Autodesk Inventor part; units mm, degrees
ref_plane "YZ Plane" through (0, 0, 0) normal (1, 0, 0) x (0, 1, 0)
ref_plane "XZ Plane" through (0, 0, 0) normal (0, 1, 0) x (-1, 0, 0)
ref_plane "XY Plane" through (0, 0, 0) normal (0, 0, 1) x (1, 0, 0)
sketch "Block1" plane through (0, 0, 0) normal (0, 0, 1) x (1, 0, 0)
  circle A0 centre (40.64, 3.81) radius 3.81
  point P0 (32.0567, 3.81)
sketch "Sketch1" plane through (0, 0, 0) normal (0, 1, 0) x (-1, 0, 0)
  line L0 (5.08, 5.08) -> (-5.08, 5.08)
  line L1 (-5.08, 5.08) -> (-5.08, -39.37)
  line L2 (-5.08, -39.37) -> (5.08, -39.37)
  line L3 (5.08, -39.37) -> (5.08, 5.08)
  point P0 (0, 0)
  dimension "d0" = 10.16
  dimension "d1" = 44.45
extrude "bar" add sketch "Sketch1" along normal blind 7.62
sketch "Sketch2" plane through (-5.08, 0, -39.37) normal (-1, 0, 0) x (0, 0, 1)
  circle A0 centre (4, 3.81) radius 2.175
  circle A1 centre (16, 3.81) radius 2.175
  circle A2 centre (9.9822, 3.81) radius 1.0704
  point P0 (39.37, 0)
  dimension "d4" = 4.35
  dimension "d5" = 4.35
hole "pegholes" at (-5.08, 3.81, -35.37) at (-5.08, 3.81, -23.37) direction (1, 0, 0) diameter 4.35 end through all
fillet "Fillet3" radius 3.81 3 edges at (0, 7.62, -39.37) (0, 0, -39.37) (0, 7.62, 5.08)
sketch "Sketch3" plane through (5.08, 0, 5.08) normal (1, 0, 0) x (0, 0, -1)
  line L0 (40.64, 7.62) -> (3.81, 7.62)
  line L1 (23.6161, 7.62) -> (40.64, 7.62)
  line L2 (40.64, 7.62) -> (40.64, 0)
  line L3 (40.64, 0) -> (23.6161, 0)
  line L4 (23.6161, 0) -> (23.6161, 7.62)
  circle A0 centre (40.64, 3.81) radius 3.81
  point P0 (5.08, 0)
extrude "Extrusion2" cut sketch "Sketch3" against normal blind 5.334 contours A0 L2 | L2 A0
extrude "Extrusion3" cut sketch "Sketch3" against normal blind 5.334 contours A0 L3 L4 L0 | L2 A0 picked at (39.3793, 3.6569)
fillet "Fillet4" radius 5.334 1 edges at (5.08, 3.81, -18.5361)
properties part number "fire-bar"
Can you work these out from the model? Positions are in its coordinate system, mm. A direction names the side the tool comes from. Coordinates: 2 decimals unless noted, no trailing zeros. Loops run counter-clockwise (first coordinate to the right, second up) from the corner with the lowest first, then second, coordinate; pieces in that order, holes last.
1) Imagine slicing it at C-C on x = 1.5. List the corners of the cut face in (y, z) for me, plus the area to 3 significant figures.
2) Thinking about a two-plate mould opening in Y: for faces 3 (the flat face through (-1, 7.62, -13)), 4 (the flat face through (-1, 0, -10)), 5 (the cylindrical face through (-2.633, 3.157, -21.295)), 6 (the flat face through (-5.08, 4, -17)), which applies, pulls with the +Y half, pulls with the -Y half, needs draft (parallel to the pull), parting line crosses it, or undercut?
3) For pin 1 (4 mm diameter, centred on y = 3.5, z = -32, fed in from +X); pin 2 (3 mm diameter, centred on x = -2, y = 5.5, fed in from -Z), each with a flat end and sliding along its axis, tell me the tip position at first contact or that it passes through.
4) Imagine slicing it at D-D on z = -29.5. List the corners of the cut face in (x, y) for me, plus the area to 3 significant figures.
5) Imagine slicing it at A-A on z = -23.37. List the corners of the cut face in (x, y) for me (3 decimals), plus the area to 3 significant figures.
6) Which directions (+Z, -Z, +X, -X, +Y, -Y) give clear straight access to the entire face, cutting with the end or side of a thin tool? Please do faces 1 (the flat face through (0, 2, 5.08)), 2 (the flat face through (-0.254, 4, -29)).
7) Imagine slicing it at B-B on x = -3.25. State how many separate pieces and enclosed holes the cut face has, plus the area to 3 significant figures.
8) I need wall thicknesses on probe 1 along Z at (x, y) = (-3.25, 3.81) (3 decimals). Which ranges of the line are inside material? Lowest first, please.
Completed:
1. outline: (0, -18.24) - (7.62, -18.24) - (7.62, 1.27) arc R3.81 ccw to (3.81, 5.08) - (0, 5.08) - close
1. area: 175 mm2
2. face 3: pulls with the +Y half
2. face 4: pulls with the -Y half
2. face 5: undercut
2. face 6: needs draft
3. pin 1: stops at x = -0.25
3. pin 2: stops at z = -39.37
4. outline: (-5.08, 0) - (-0.25, 0) - (-0.25, 7.62) - (-5.08, 7.62) - close
4. area: 36.8 mm2
5. outline: (-5.08, 0) - (-0.254, 0) - (-0.254, 1.635) - (-5.08, 1.635) - close; (-5.08, 5.985) - (-0.254, 5.985) - (-0.254, 7.62) - (-5.08, 7.62) - close
5. area: 15.8 mm2
6. face 1: +Z, +X, -X, +Y, -Y
6. face 2: -Z, +X, +Y, -Y
7. separate pieces: 1
7. enclosed holes: 2
7. area: 300 mm2
8. probe 1: z = -39.37 to -37.545, -33.195 to -25.545, -21.195 to 5.08
